Build history of the part. All positions in model axes, mm. A direction names the side the tool comes from. Round coordinates to 2 decimals unless told otherwise and drop trailing zeros. Write each loop counter-clockwise with the first axis right and the second up, starting at its lowest first coordinate (ties: lowest second). Pieces come first, ordered by that corner, then holes. Notation, with made-up numbers: (53.5, 14.5) -> (99.5, 14.5) arc R8 cw to (99.5, 29.5) -> close; hole circle Ø10 at (17, 21.25). An arc over 180 degrees is marked (long way). One line per question, with ' | ' between items.
from build123d import *

# Parameters (mm, degrees)
SKETCH1_W           = 45
SKETCH1_H           = 52
BOSS_EXTRUDE1_DEPTH = 3
SKETCH2_W           = 35
SKETCH2_H           = 42
BOSS_EXTRUDE2_DEPTH = 4
SKETCH3_W           = 15
SKETCH3_H           = 6
CUT_EXTRUDE1_DEPTH  = 70.123078635
FILLET1_R           = 3


with BuildPart() as part:
    # Sketch1 → Boss-Extrude1 (new body)
    with BuildSketch(Plane.XY):
        with Locations((22.5, 26)):
            Rectangle(SKETCH1_W, SKETCH1_H)
    extrude(amount=BOSS_EXTRUDE1_DEPTH)

    # Sketch2 → Boss-Extrude2 (add)
    with BuildSketch(Plane.XY.offset(3)):
        with Locations((22.5, 26)):
            Rectangle(SKETCH2_W, SKETCH2_H)
    extrude(amount=BOSS_EXTRUDE2_DEPTH)

    # Sketch3 → Cut-Extrude1 (cut, through all)
    with BuildSketch(Plane.XY.offset(7)):
        with Locations((22.5, 13)):
            Rectangle(SKETCH3_W, SKETCH3_H)
    extrude(amount=-CUT_EXTRUDE1_DEPTH, mode=Mode.SUBTRACT)

    # Fillet1
    fillet1_edges = [part.edges().sort_by_distance(p)[0] for p in [
        (30, 10, 3.5),
        (15, 10, 3.5),
        (30, 16, 3.5),
        (15, 16, 3.5),
        (45, 0, 1.5),
        (0, 0, 1.5),
    ]]
    fillet(fillet1_edges, radius=FILLET1_R - 0.0001)  # a hair under: the kernel refuses the full size


solid = part.part
(1) Drop flat-ended pins along their axis: pin 1 (2 mm diameter, centred on x = 27, z = 6, fed in from +Y); pin 2 (1.2 mm diameter, centred on y = 29, z = 5.5, fed in from +X); pin 3 (4 mm diameter, centred on x = 14, z = 5.5, fed in from -Y). Give the stop position or say it passes through.
Calculated:
pin 1: y = 47 | pin 2: x = 40 | pin 3: y = 5
(2) Slice it at C-C (y = 22.5). Write the cut outline in (x, z), then the cut area to 3 significant figures.
Calculated:
outline: (0, 0) -> (45, 0) -> (45, 3) -> (40, 3) -> (40, 7) -> (5, 7) -> (5, 3) -> (0, 3) -> close | area: 275 mm2
(3) 3-axis set-ups, long thin cutter, end or side, ignore diameter. For faces 4 (the flat face through (22, 47, 5)), 5 (the flat face through (40, 26, 5)), 6 (the cylindrical face through (29.1, 10.86, 3.45)): which of +Z, -Z, +X, -X, +Y, -Y reach the whole face in a straight line?
Calculated:
face 4: +Z, +X, -X, +Y | face 5: +Z, +X, +Y, -Y | face 6: +Z, -Z
(4) Wall check: line 1 (Y direction, x = 13, z = 5.5); line 2 (X direction, y = 27, z = 4.5); line 3 (X direction, y = 12, z = 5.25). Give the ranges that are in metal, low to high. Write a range as from..to.
Calculated:
line 1: 5..47 | line 2: 5..40 | line 3: 5..15.17, 29.83..40
(5) Slice it at B-B (x = 33). Write the cut outline in (y, z), then the cut area to 3 significant figures.
Calculated:
outline: (0, 0) -> (52, 0) -> (52, 3) -> (47, 3) -> (47, 7) -> (5, 7) -> (5, 3) -> (0, 3) -> close | area: 324 mm2
(6) Mould opens along X. For faces 1 (the flat face through (0, 27, 1)), 2 (the cylindrical face through (15.9, 15.14, 3.45)), 3 (the flat face through (22, 52, 1)) say: pulls with the +X half, pulls with the -X half, needs draft (parallel to the pull), parting line crosses it, or undercut.
Calculated:
face 1: pulls with the -X half | face 2: undercut | face 3: needs draft
